Answer from the drawing. Dimensions are ordinates in mm from the lowest x, y and z of the part. Coordinates: 2 decimals unless noted, no trailing zeros. Order: outer loops, then holes, each group sorted by start corner. A loop starts at its lowest first (then second) coordinate and runs counter-clockwise, first axis right, second up. Notation, with made-up numbers: (79.5, -11.75) - (130.5, -11.75) arc R18 ccw to (130.5, 13.25) - close; hole circle Ø2 at (-3.75, -15). An arc over 180 degrees is marked (long way). Use a Markdown table: item, result. Add a question column.
Item 1: Find the intervals of material crossed by line 1 along X through (y, z) = (25, 4.75) (3 decimals); line 2 along X through (y, z) = (111, 5.75); line 3 along Y through (x, z) = (168, 6.5), in increasing order.
Item 2: The part is cut by section A-A, the plane z = 10.75. Give the vertices of the cut face in (x, y) (3 decimals), then the cut area to 3 significant figures.
Item 3: A flat-ended cylindrical pin translates along its axis: P1, Ø8, axis at x = 114, y = 111, coming from the +Z side. Find the tip coordinate at first contact, or state that the pin passes through.
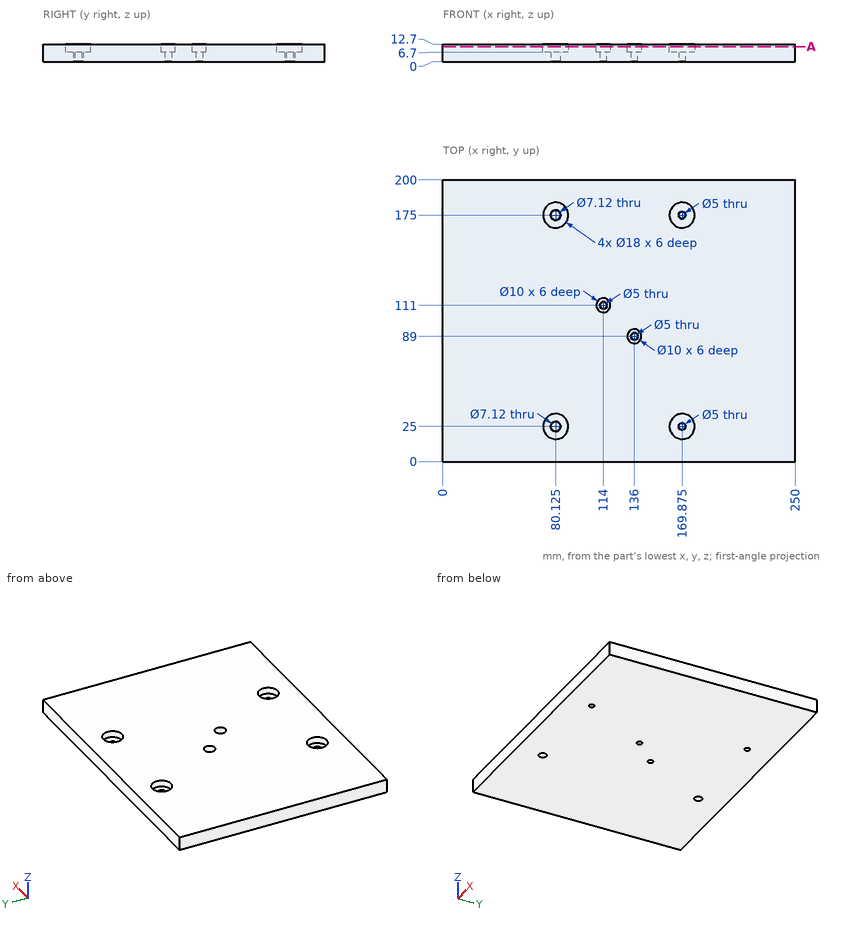
Solution:
| question | item | result |
|---|---|---|
| 1 | line 1 | x = 0 to 76.565, 83.685 to 167.375, 172.375 to 250 |
| 1 | line 2 | x = 0 to 111.5, 116.5 to 250 |
| 1 | line 3 | y = 0 to 23.35, 26.65 to 173.35, 176.65 to 200 |
| 2 | outline | (0, 0) - (250, 0) - (250, 200) - (0, 200) - close; hole circle Ø18 at (80.125, 25); hole circle Ø18 at (80.125, 175); hole circle Ø10 at (114, 111); hole circle Ø10 at (136, 89); hole circle Ø18 at (169.875, 25); hole circle Ø18 at (169.875, 175) |
| 2 | area | 48,800 mm2 |
| 3 | P1 | stops at z = 6.7 |
